Answer from the drawing. Dimensions are ordinates in mm from the lowest x, y and z of the part. A direction names the side the tool comes from. Round coordinates to 2 decimals unless told otherwise and drop trailing zeros. Order: outer loops, then holes, each group sorted by start corner. A loop starts at its lowest first (then second) coordinate and runs counter-clockwise, first axis right, second up.
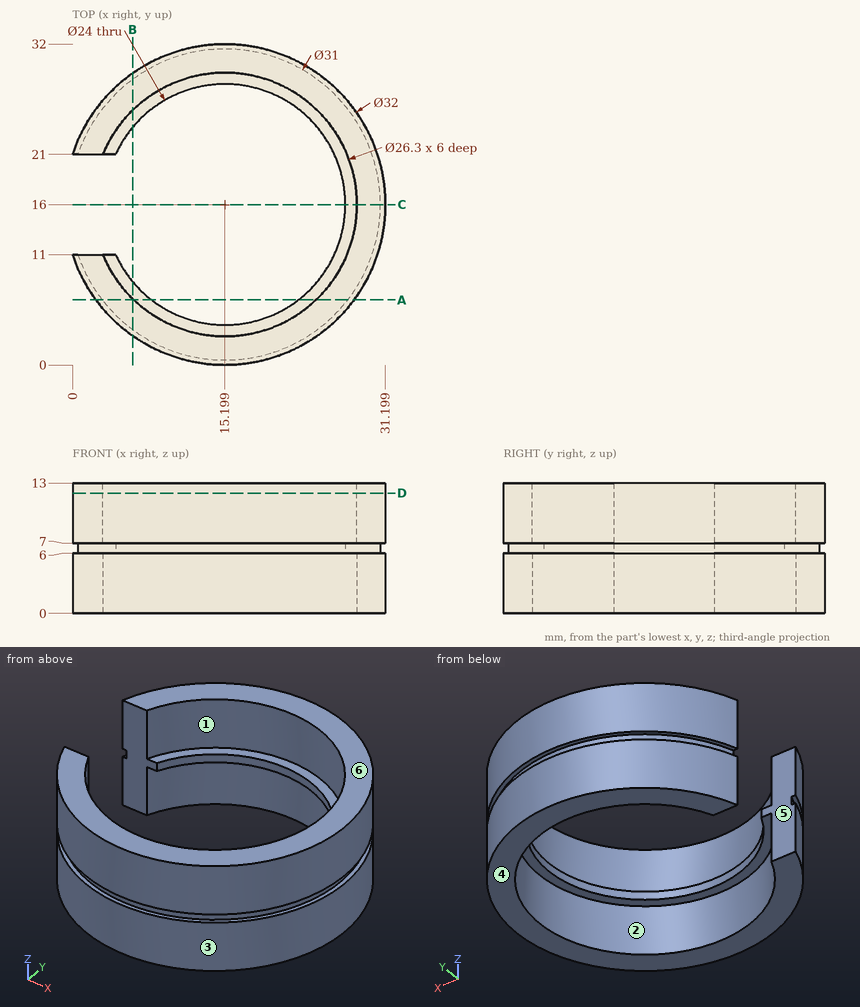
Q1. For the marked faces 5 and 6, determine the directions among +Z, -Z, +X, -X, +Y, -Y from which every point of the face is accessible in a straight line to the end or side of a thin tool.
Outcome:
face 5: +Z, -Z, -X
face 6: +Z, +X, -X, +Y, -Y
Q2. A cutting plane is placed at A-A, the plane y = 6.5. Give the vertices of the cut face in (x, z).
Outcome:
outline: (2.32, 0) - (6.11, 0) - (6.11, 6) - (7.87, 6) - (7.87, 7) - (6.11, 7) - (6.11, 13) - (2.32, 13) - (2.32, 7) - (2.95, 7) - (2.95, 6) - (2.32, 6) - close; (22.53, 6) - (24.29, 6) - (24.29, 0) - (28.07, 0) - (28.07, 6) - (27.45, 6) - (27.45, 7) - (28.07, 7) - (28.07, 13) - (24.29, 13) - (24.29, 7) - (22.53, 7) - close
Q3. Straight lines are drawn through the part: probe 1 along Y at (x, z) = (22, 0.75) (1 decimal); probe 2 along X at (y, z) = (25, 10) (1 decimal); probe 3 along X at (y, z) = (16, 10.65). For each, find the intervals that lie inside material, in ascending order.
Outcome:
probe 1: y = 1.5 to 4.7, 27.3 to 30.5
probe 2: x = 2 to 5.6, 24.8 to 28.4
probe 3: x = 28.35 to 31.2
Q4. For a pull along X with two mould halves and no side action, classify the marked faces 1, 2, 3 and 4 as released by +X, released by -X, zero draft, split by the parting line, or undercut.
Outcome:
face 1: undercut
face 2: undercut
face 3: split by the parting line
face 4: zero draft
Q5. A cutting plane is placed at C-C, the plane y = 16. Give the vertices of the cut face in (x, z), plus the area to 3 significant figures.
Outcome:
outline: (27.2, 6) - (28.35, 6) - (28.35, 0) - (31.2, 0) - (31.2, 6) - (30.7, 6) - (30.7, 7) - (31.2, 7) - (31.2, 13) - (28.35, 13) - (28.35, 7) - (27.2, 7) - close
area: 37.7 mm2
Q6. A cutting plane is placed at D-D, the plane z = 12. Give the vertices of the cut face in (x, y).
Outcome:
outline: (0, 11) arc R16 ccw (long way) to (0, 21) - (3.04, 21) arc R13.15 cw (long way) to (3.04, 11) - close
Q7. A cutting plane is placed at B-B, the plane x = 6. Give the vertices of the cut face in (y, z) (1 decimal), plus the area to 3 significant figures.
Outcome:
outline: (2.9, 0) - (6.6, 0) - (6.6, 6) - (8.3, 6) - (8.3, 7) - (6.6, 7) - (6.6, 13) - (2.9, 13) - (2.9, 7) - (3.5, 7) - (3.5, 6) - (2.9, 6) - close; (23.7, 6) - (25.4, 6) - (25.4, 0) - (29.1, 0) - (29.1, 6) - (28.5, 6) - (28.5, 7) - (29.1, 7) - (29.1, 13) - (25.4, 13) - (25.4, 7) - (23.7, 7) - close
area: 98.2 mm2
Q8. Flat-ended cylindrical pins translate along their axes: pin 1 (1.5 mm diameter, centred on y = 18.5, z = 10, fed in from +X); pin 2 (3.5 mm diameter, centred on x = 2.5, z = 5.5, fed in from +Y); pin 3 (4.5 mm diameter, centred on x = 3, z = 7, fed in from -Y). Find the tip coordinate at first contact, or state that the pin passes through.
Outcome:
pin 1: stops at x = 31.1
pin 2: stops at y = 27.67
pin 3: stops at y = 3.47
